Can you work these out from the model? Positions are in its coordinate system, mm. A direction names the side the tool comes from. Coordinates: 2 decimals unless noted, no trailing zeros. Order: outer loops, then holes, each group sorted by start corner. A loop starts at its lowest first (then second) coordinate and runs counter-clockwise, first axis right, second up. Notation, with made-up numbers: (51, 70.25) - (84, 70.25) arc R7 cw to (84, 77.25) - close; hole circle Ø1 at (16, -10.5). An arc over 180 degrees is marked (long way). Return JSON: item names as keys, results as strings. Group by question number.
1) Imagine slicing it at A-A (x = -16.7). Write out the boundary of the cut face in (y, z), and give its area (3 significant figures).
2) If we mould it in two halves opening along X, with no side actions, what happens to faces 4 (the face through (-40, 4, 0)), 5 (the face through (40, 4, 0)), 6 (the face through (28.53, 1.48, 5.5))? For each: pulls with the +X half, pulls with the -X half, needs draft (parallel to the pull), parting line crosses it, or undercut.
3) Imagine slicing it at B-B (z = -3.25). Write out the boundary of the cut face in (x, y), and give its area (3 significant figures).
4) Imagine slicing it at D-D (z = 3). Give the number of separate pieces and of enclosed holes in the cut face, and give its area (3 significant figures).
5) Imagine slicing it at C-C (y = 7). Write out the boundary of the cut face in (x, z), and give its area (3 significant figures).
6) Which directions (+Z, -Z, +X, -X, +Y, -Y) give clear straight access to the entire face, cutting with the end or side of a thin tool? Please do faces 1 (the face through (1, 0, 0)), 2 (the face through (-28.53, 1.48, 0.5)), 3 (the face through (14, 4, 0)).
7) If I drill on line 1 along X through (y, z) = (4.5, 3); line 2 along X through (y, z) = (6, 5.25); line 3 along X through (y, z) = (0.5, 3.75), over which ranges is the centre line in solid material (lowest first)?
8) For pin 1 Ø8 at (x, z) = (-21.5, 0.5) entering from +Y; pin 2 Ø2.5 at (x, z) = (-30, 3) entering from -Y; pin 3 Ø3 at (x, z) = (-30, 4.5) entering from -Y, each with a flat end and sliding along its axis, tell me the tip position at first contact or that it passes through.
Autodesk Inventor part; units mm, degrees
ref_plane "YZ Plane" through (0, 0, 0) normal (1, 0, 0) x (0, 1, 0)
ref_plane "XZ Plane" through (0, 0, 0) normal (0, 1, 0) x (-1, 0, 0)
ref_plane "XY Plane" through (0, 0, 0) normal (0, 0, 1) x (1, 0, 0)
sketch "Boceto1" plane through (0, 0, 0) normal (0, 1, 0) x (-1, 0, 0)
  line L0 (-40, 8) -> (40, 8)
  line L1 (40, 8) -> (40, -8)
  line L2 (40, -8) -> (-40, -8)
  line L3 (-40, -8) -> (-40, 8)
  line L4 (-40, 8) -> (40, -8) construction
  line L5 (40, 8) -> (-40, -8) construction
  circle A0 centre (-16.7, 4) radius 2.7
  circle A1 centre (-16.7, -4) radius 2.7
  circle A2 centre (16.7, 4) radius 2.7
  circle A3 centre (16.7, -4) radius 2.7
  line L6 (19.4, 4) -> (14, 4)
  line L7 (14, 4) -> (14, -4)
  line L8 (14, -4) -> (19.4, -4)
  line L9 (19.4, -4) -> (19.4, 4)
  line L10 (-14, 4) -> (-19.4, 4)
  line L11 (-19.4, 4) -> (-19.4, -4)
  line L12 (-19.4, -4) -> (-14, -4)
  line L13 (-14, -4) -> (-14, 4)
  point P0 (0, 0)
  point P1 (16.7, -4)
  point P2 (16.7, 4)
  point P3 (-16.7, -4)
  point P4 (-16.7, 4)
  point P5 (19.4, -4)
  point P6 (-14, -4)
  point P7 (-19.4, -4)
  point P8 (-19.4, 4)
  dimension "d2" = 5.4
  dimension "d0" = 80
  dimension "d1" = 16
  dimension "d3" = 4
  dimension "d4" = 8
  dimension "d5" = 23.3
  dimension "d35" = 23.3
extrude "Extrusión1" add sketch "Boceto1" along normal blind 8
fillet "Empalme2" radius 3 4 edges at (-40, 4, 8) (-40, 4, -8) (40, 4, 8) (40, 4, -8)
sketch "Boceto6" plane through (0, 8, 0) normal (0, 1, 0) x (1, 0, 0)
  circle A0 centre (-30, -3) radius 1.65
  circle A1 centre (30, -3) radius 1.65
  line L0 (37, 8) -> (-37, 8)
  line L1 (30, -3) -> (-30, -3)
  line L2 (-37, -8) -> (37, -8)
  point P0 (0, 0)
  dimension "d27" = 3.3
  dimension "d48" = 11
  dimension "d51" = 60
  dimension "d52" = 30
extrude "Extrusión6" cut sketch "Boceto6" against normal through all
sketch "Boceto11" plane through (0, 0, 0) normal (0, -1, 0) x (1, 0, 0)
  circle A0 centre (-30, 3) radius 1.65
  circle A1 centre (-30, 3) radius 2.9
  circle A2 centre (30, 3) radius 1.65
  circle A3 centre (30, 3) radius 2.9
  line L0 (-32.9, 4.6743) -> (-30, 6.3486)
  line L1 (-30, 6.3486) -> (-27.1, 4.6743)
  line L2 (-27.1, 4.6743) -> (-27.1, 1.3257)
  line L3 (-27.1, 1.3257) -> (-30, -0.3486)
  line L4 (-30, -0.3486) -> (-32.9, 1.3257)
  line L5 (-32.9, 1.3257) -> (-32.9, 4.6743)
  line L6 (30, -0.3486) -> (27.1, 1.3257)
  line L7 (27.1, 1.3257) -> (27.1, 4.6743)
  line L8 (27.1, 4.6743) -> (30, 6.3486)
  line L9 (30, 6.3486) -> (32.9, 4.6743)
  line L10 (32.9, 4.6743) -> (32.9, 1.3257)
  line L11 (32.9, 1.3257) -> (30, -0.3486)
  point P0 (0, 0)
  dimension "d45" = 5.8
extrude "Extrusión10" cut sketch "Boceto11" against normal blind 3 contours A0 | A1 | L2 L3 A1 | A1 L1 L2 | A1 L0 L1 | L3 L4 A1 | A1 L5 L0 | L4 L5 A1 | A2 | A3 | L10 L11 A3 | A3 L9 L10 | A3 L8 L9 | L11 L6 A3 | A3 L7 L8 | L6 L7 A3
sketch "Boceto12" plane through (0, 8, 0) normal (0, 1, 0) x (1, 0, 0)
  circle A0 centre (-30, -3) radius 1.65
  circle A1 centre (-30, -3) radius 2.375
  circle A2 centre (30, -3) radius 1.65
  circle A3 centre (30, -3) radius 2.375
  point P0 (0, 0)
  dimension "d53" = 4.75
  dimension "d54" = 4.75
extrude "Extrusión11" add sketch "Boceto12" along normal blind 1.4
fillet "Empalme3" radius 1.4 2 edges at (-32.375, 8, 3) (27.625, 8, 3)
sketch "Boceto5" plane through (0, 0, 0) normal (0, -1, 0) x (1, 0, 0)
  circle A0 centre (-30, -4.1) radius 1.7
  circle A1 centre (-30, -4.1) radius 2.875
  circle A2 centre (20, -4.1) radius 1.7
  circle A3 centre (20, -4.1) radius 2.875
  line L0 (-33.3198, -4.1) -> (-31.6599, -1.225)
  line L1 (-31.6599, -1.225) -> (-28.3401, -1.225)
  line L2 (-28.3401, -1.225) -> (-26.6802, -4.1)
  line L3 (-26.6802, -4.1) -> (-28.3401, -6.975)
  line L4 (-28.3401, -6.975) -> (-31.6599, -6.975)
  line L5 (-31.6599, -6.975) -> (-33.3198, -4.1)
  line L6 (16.6802, -4.1) -> (18.3401, -1.225)
  line L7 (18.3401, -1.225) -> (21.6599, -1.225)
  line L8 (21.6599, -1.225) -> (23.3198, -4.1)
  line L9 (23.3198, -4.1) -> (21.6599, -6.975)
  line L10 (21.6599, -6.975) -> (18.3401, -6.975)
  line L11 (18.3401, -6.975) -> (16.6802, -4.1)
  point P0 (0, 0)
  dimension "d24" = 5.75
properties part number "Rack support"
Calculated:
{
 "1": {"outline": "(0, -8) - (8, -8) - (8, -6.7) - (0, -6.7) - close; (0, 6.7) - (8, 6.7) - (8, 8) - (0, 8) - close", "area": "20.8 mm2"},
 "2": {"face 4": "pulls with the -X half", "face 5": "pulls with the +X half", "face 6": "undercut"},
 "3": {"outline": "(-40, 0) - (-19.4, 0) - (-19.4, 8) - (-40, 8) - close; (-14, 0) - (14, 0) - (14, 8) - (-14, 8) - close; (19.4, 0) - (40, 0) - (40, 8) - (19.4, 8) - close", "area": "554 mm2"},
 "4": {"separate pieces": "5", "enclosed holes": "0", "area": "492 mm2"},
 "5": {"outline": "(-40, -5) arc R3 ccw to (-37, -8) - (37, -8) arc R3 ccw to (40, -5) - (40, 5) arc R3 ccw to (37, 8) - (-37, 8) arc R3 ccw to (-40, 5) - close; hole circle Ø3.3 at (-30, 3); hole (-19.4, -4) arc R2.7 ccw to (-14, -4) - (-14, 4) arc R2.7 ccw to (-19.4, 4) - close; hole (14, -4) arc R2.7 ccw to (19.4, -4) - (19.4, 4) arc R2.7 ccw to (14, 4) - close; hole circle Ø3.3 at (30, 3)", "area": "1,120 mm2"},
 "6": {"face 1": "+Z, -Z, +X, -X, -Y", "face 2": "-Y", "face 3": "+Y, -Y"},
 "7": {"line 1": "-40 to -31.65, -28.35 to -19.4, -14 to 14, 19.4 to 28.35, 31.65 to 40", "line 2": "-39.99 to -19.09, -14.31 to 14.31, 19.09 to 39.99", "line 3": "-40 to -32.9, -27.1 to -19.4, -14 to 14, 19.4 to 27.1, 32.9 to 40"},
 "8": {"pin 1": "y = 8", "pin 2": "through", "pin 3": "y = 3"}
}
